Check sheet for the modelled part. Datum: model origin and axes. Units: mm. Round coordinates to 2 decimals unless told otherwise and drop trailing zeros. Write each loop counter-clockwise with the first axis right and the second up, starting at its lowest first coordinate (ties: lowest second). Pieces come first, ordered by that corner, then holes.
Item 1: Release check for a two-part mould opening along X. For faces 1 (the flat face through (0, 0, 2)), 2 (the cylindrical face through (-0.2, 3.54, -1.51)) record: pulls with the +X half, pulls with the -X half, needs draft (parallel to the pull), parting line crosses it, or undercut.
Item 2: Material ranges on line 1 along Y through (x, z) = (1.6, 1.45) (3 decimals); line 2 along Y through (x, z) = (-1.8, -1) (3 decimals); line 3 along Z through (x, y) = (0.15, 1), recorded low to high.
Item 3: Section check B-B, the plane y = 0.5. Record the cut outline in (x, z), plus the area to 3 significant figures.
Item 4: Section check A-A, the plane y = 4. Record the cut outline in (x, z), plus the area to 3 significant figures.
Item 5: Depth check by flat-ended pin: pin 1 (2 mm diameter, centred on x = -0.5, y = 1, fed in from +Z). Enter the tip coordinate at first touch or a pass-through.
from build123d import *

# Parameters (mm, degrees)
FILLET1_R = 0.508
FILLET2_R = 0.0762


with BuildPart() as part:
    # Sketch1 → Revolve1 (revolve)
    with BuildSketch(Plane.XY):
        with BuildLine():
            Line((1.524, 0), (1.524, 6.985))
            Line((1.524, 6.985), (2.4892, 6.985))
            Line((2.4892, 6.985), (1.777274138, 5.7785))
            ThreePointArc((1.777274138, 5.7785), (2.8956, 3.4925), (1.777274138, 1.2065))
            Line((1.777274138, 1.2065), (2.4892, 0))
            Line((2.4892, 0), (1.524, 0))
        make_face()
    revolve(axis=Axis((0, 0, 0), (0, 1, 0)))

    # Fillet1
    fillet1_edges = [part.edges().sort_by_distance(p)[0] for p in [
        (-1.777274138, 1.2065, 0),
        (-1.777274138, 5.7785, 0),
    ]]
    fillet(fillet1_edges, radius=FILLET1_R)

    # Fillet2
    fillet2_edges = [part.edges().sort_by_distance(p)[0] for p in [
        (-2.4892, 0, 0),
        (-2.4892, 6.985, 0),
    ]]
    fillet(fillet2_edges, radius=FILLET2_R)


solid = part.part
Values found:
1. face 1: needs draft
1. face 2: undercut
2. line 1: y = 0 to 0.559, 1.563 to 5.422, 6.426 to 6.985
2. line 2: y = 0 to 0.729, 1.457 to 5.528, 6.256 to 6.985
2. line 3: z = -1.92 to -1.52, 1.52 to 1.92
3. outline: circle Ø4.39 at (0, 0); hole circle Ø3.05 at (0, 0)
3. area: 7.83 mm2
4. outline: circle Ø5.7 at (0, 0); hole circle Ø3.05 at (0, 0)
4. area: 18.2 mm2
5. pin 1: stops at z = 2.45
